Source: CAD feature listing. Evaluate the final solid. Frame: model axes, mm. Face numbers are marked on the shaded views. A direction names the side the tool comes from. Give positions to 0.01 mm unless a question says otherwise; leave off trailing zeros. Loops run counter-clockwise (first coordinate to the right, second up) from the corner with the lowest first, then second, coordinate; pieces in that order, holes last.
Autodesk Inventor part; units mm, degrees
ref_plane "YZ Plane" through (0, 0, 0) normal (1, 0, 0) x (0, 1, 0)
ref_plane "XZ Plane" through (0, 0, 0) normal (0, 1, 0) x (-1, 0, 0)
ref_plane "XY Plane" through (0, 0, 0) normal (0, 0, 1) x (1, 0, 0)
sketch "Sketch1" plane through (0, 0, 0) normal (0, 0, 1) x (1, 0, 0)
  circle A0 centre (0, 0) radius 4.7625
  dimension "d0" = 9.525
extrude "Extrusion1" add sketch "Sketch1" along normal blind 15.24
sketch "Sketch2" plane through (0, 0, 15.24) normal (0, 0, 1) x (1, 0, 0)
  circle A0 centre (0, 0) radius 6.096
  dimension "d3" = 12.192
extrude "Extrusion2" add sketch "Sketch2" along normal blind 44.45
sketch "Sketch3" plane through (0, 0, 59.69) normal (0, 0, 1) x (1, 0, 0)
  circle A0 centre (0, 0) radius 12.7
  dimension "d7" = 25.4
loft "Loft1" add profiles "Sketch3" section 2 edges at (-6.096, 0, 15.24)
sketch "Sketch4" plane through (0, 0, 59.69) normal (0, 0, 1) x (1, 0, 0)
  circle A0 centre (0, 0) radius 12.7
extrude "Extrusion3" add sketch "Sketch4" along normal blind 19.05
chamfer "Chamfer1" distance 1.143 angle 45 1 edges at (-12.7, 0, 78.74)
properties part number "JB_CAD_FinalPt2"
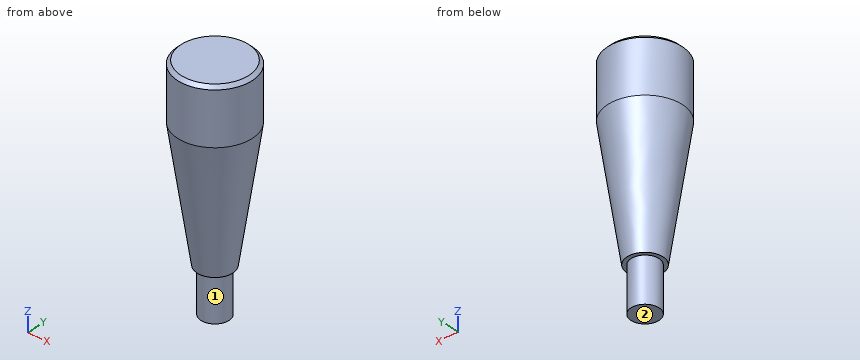
(1) Section C-C, the plane z = 72. Return the cut outline in (x, y), then the cut area to 3 significant figures.
A:
outline: circle Ø25.4 at (0, 0)
area: 507 mm2
(2) Section B-B, the plane z = 52. Return the cut outline in (x, y), then the cut area to 3 significant figures.
A:
outline: circle Ø23.11 at (0, 0)
area: 420 mm2
(3) First-contact query: pin 1 (1 mm diameter, centred on x = 5, y = -3.5, fed in from -Z); pin 2 (1 mm diameter, centred on x = 3, z = 14, fed in from -Y); pin 3 (1 mm diameter, centred on y = -0.5, z = 48.5, fed in from +X). Flat tips, straight axial feed; report the tip coordinate or a pass-through.
A:
pin 1: stops at z = 15.24
pin 2: stops at y = -4.05
pin 3: stops at x = 11.1
(4) Ray query, line 1 along Z through (x, y) = (5.75, 0.75); line 2 along Y through (x, z) = (-5.5, 55); line 3 along Y through (x, z) = (-1.75, 63.5). Return the intervals inside material, ascending.
A:
line 1: z = 15.24 to 78.74
line 2: y = -10.67 to 10.67
line 3: y = -12.58 to 12.58
(5) Section A-A, the plane x = 0. Return the cut outline in (y, z), then the cut area to 3 significant figures.
A:
outline: (-12.7, 59.69) - (-6.1, 15.24) - (-4.76, 15.24) - (-4.76, 0) - (4.76, 0) - (4.76, 15.24) - (6.1, 15.24) - (12.7, 59.69) - (12.7, 77.6) - (11.56, 78.74) - (-11.56, 78.74) - (-12.7, 77.6) - close
area: 1,460 mm2
(6) Reachability of the marked faces 1 and 2 from +Z, -Z, +X, -X, +Y, -Y: full face, straight path, thin tool, end or side. Return the list, or none.
A:
face 1: -Z
face 2: -Z, +X, -X, +Y, -Y
